Geometry: final body of the model. Coordinates: model frame, mm. Face numbers are marked on the shaded views. A direction names the side the tool comes from. Give positions to 0.01 mm unless a question says otherwise; leave off trailing zeros. Loops run counter-clockwise (first coordinate to the right, second up) from the corner with the lowest first, then second, coordinate; pieces in that order, holes last.
from build123d import *

# Parameters (mm, degrees)
SKETCH1_R           = 2
BOSS_EXTRUDE1_DEPTH = 5
FILLET2_R           = 3


with BuildPart() as part:
    # Sketch1 → Boss-Extrude1 (new body)
    with BuildSketch(Plane(origin=(0, 0, 0), x_dir=(1, 0, 0), z_dir=(0, 1, 0))):
        with BuildLine():
            Line((12.081978252, 23.920233872), (28.081978252, -7.602676631))
            ThreePointArc((28.081978252, -7.602676631), (36.081978252, -15.602676631), (44.081978252, -7.602676631))
            Line((44.081978252, -7.602676631), (60.081978252, 23.920233872))
            Line((60.081978252, 23.920233872), (60.081978252, 39.133054542))
            Line((60.081978252, 39.133054542), (60.081978252, 42.765188956))
            Line((60.081978252, 42.765188956), (60.081978252, 46.397323369))
            ThreePointArc((60.081978252, 46.397323369), (52.081978252, 54.397323369), (44.081978252, 46.397323369))
            Line((44.081978252, 46.397323369), (40.081978252, 42.397323369))
            Line((40.081978252, 42.397323369), (32.081978252, 42.397323369))
            Line((32.081978252, 42.397323369), (28.081978252, 46.397323369))
            ThreePointArc((28.081978252, 46.397323369), (20.081978252, 54.397323369), (12.081978252, 46.397323369))
            Line((12.081978252, 46.397323369), (12.081978252, 39.746064801))
            Line((12.081978252, 39.746064801), (12.081978252, 23.920233872))
        make_face()
        with Locations(Location((36.081978252, -7.602676631, 0), (0, 0, 270))):
            Circle(SKETCH1_R, mode=Mode.SUBTRACT)
        Polygon((22.081978252, 19.123105702), (22.081978252, 38.397323369), (50.081978252, 38.397323369), (50.081978252, 19.123105702), (41.081978252, 8.397323369), (36.081978252, 8.397323369), (31.081978252, 8.397323369), align=None, mode=Mode.SUBTRACT)
        with Locations(Location((20.081978252, 46.397323369, 0), (0, 0, 270))):
            Circle(SKETCH1_R, mode=Mode.SUBTRACT)
        with Locations(Location((52.081978252, 46.397323369, 0), (0, 0, 270))):
            Circle(SKETCH1_R, mode=Mode.SUBTRACT)
    extrude(amount=BOSS_EXTRUDE1_DEPTH)

    # Fillet2
    fillet2_edges = [part.edges().sort_by_distance(p)[0] for p in [
        (12.081978252, 5, -35.158778621),
        (20.081978252, 5, -8.158778621),
        (36.081978252, 5, 15.602676631),
        (52.081978252, 5, -8.158778621),
        (60.081978252, 5, -35.158778621),
        (52.081978252, 5, -54.397323369),
        (42.081978252, 5, -44.397323369),
        (36.081978252, 5, -42.397323369),
        (30.081978252, 5, -44.397323369),
        (20.081978252, 5, -54.397323369),
    ]]
    fillet(fillet2_edges, radius=FILLET2_R)


solid = part.part
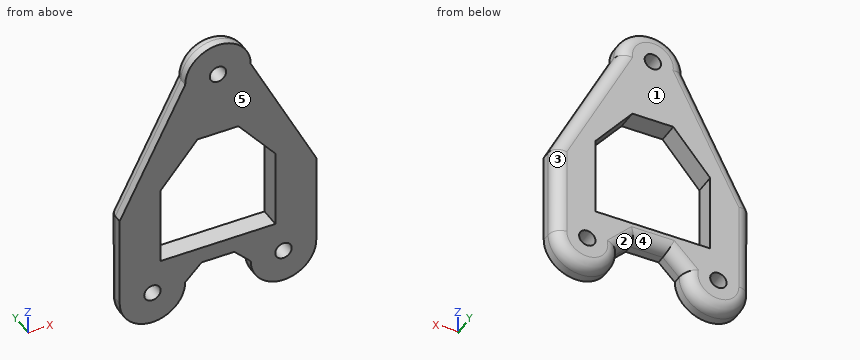
Item 1: Draft query along X for the marked faces 1, 2 and 3. Return one class per face: +X half, -X half, draft (parallel to the pull), parting line (faces both ways), or undercut.
Values follow:
face 1: draft
face 2: undercut
face 3: +X half
Item 2: Set-up query: the marked faces 4 and 5. Return all of +Z, -Z, +X, -X, +Y, -Y with unobstructed straight access to the full face (end or side cutting, diameter ignored); none if empty.
Values follow:
face 4: -Z, +Y
face 5: +Z, -Z, +X, -X, -Y
Item 3: Section query A-A on y = 1.25. Return loops of the section in (x, z), plus the area to 3 significant figures.
Values follow:
outline: (12.08, -46.4) arc R8 ccw to (28.08, -46.4) - (32.08, -42.4) - (40.08, -42.4) - (44.08, -46.4) arc R8 ccw to (60.08, -46.4) - (60.08, -23.92) - (44.08, 7.6) arc R8 ccw to (28.08, 7.6) - (12.08, -23.92) - close; hole circle Ø4 at (20.08, -46.4); hole (22.08, -38.4) - (50.08, -38.4) - (50.08, -19.12) - (41.08, -8.4) - (31.08, -8.4) - (22.08, -19.12) - close; hole circle Ø4 at (36.08, 7.6); hole circle Ø4 at (52.08, -46.4)
area: 1,560 mm2
Item 4: Ray query, probe 1 along X at (y, z) = (2.2, -28); probe 2 along Z at (x, y) = (37.5, 3.45); probe 3 along X at (y, z) = (0.4, -18). Return the intervals inside material, ascending.
Values follow:
probe 1: x = 12.09 to 22.08, 50.08 to 60.08
probe 2: z = -42.02 to -38.4, -8.4 to 6.19, 9.01 to 15.1
probe 3: x = 15.09 to 23.02, 49.14 to 57.08
Item 5: Section query B-B on x = 35. Give the number of separate pieces and of enclosed holes in the cut face, plus the area to 3 significant figures.
Values follow:
separate pieces: 3
enclosed holes: 0
area: 119 mm2
Item 6: Pin query (flat end, axial travel): pin 1 (3 mm diameter, centred on x = 28.5, y = 3, fed in from -Z); pin 2 (1.6 mm diameter, centred on x = 36, y = 0.5, fed in from -Z); pin 3 (3 mm diameter, centred on y = 1, z = -16, fed in from -X). Return the tip coordinate at first contact, or that it passes through.
Values follow:
pin 1: stops at z = -50.2
pin 2: stops at z = -42.4
pin 3: stops at x = 15.34
